Could you check a few things on this drawing? It's one solid part, dimensions in mm from its lowest x, y, z. A direction names the side the tool comes from. Give positions to 0.01 mm unless a question says otherwise; leave off trailing zeros. Loops run counter-clockwise (first coordinate to the right, second up) from the corner with the lowest first, then second, coordinate; pieces in that order, holes last. Notation, with made-up numbers: M -39.75,-10.5 L 4.25,-10.5 A11 ccw 4.25,9.5 Z; hole C -12,22 d4. An arc over 180 degrees is marked long. Answer as a JSON object with one key per item and string values.
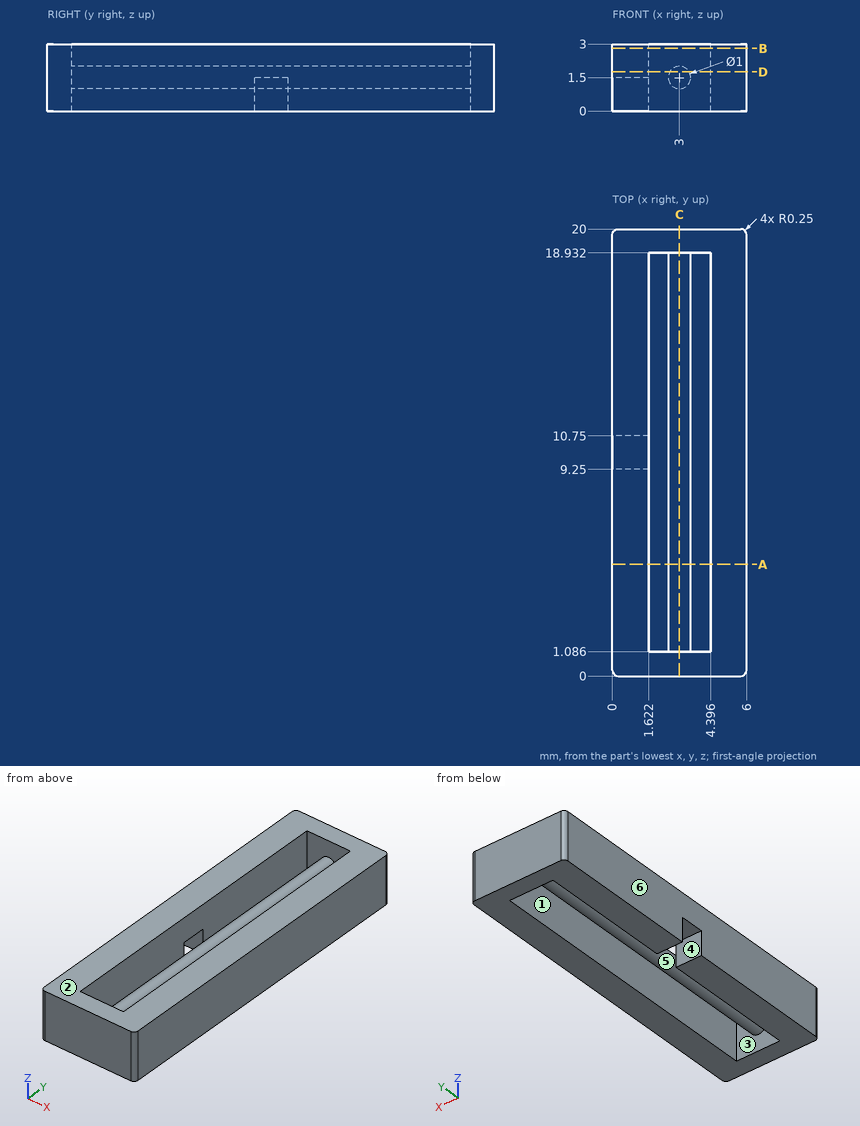
1) Suppose I cut it at C-C, the plane x = 3. Write out the boundary of the cut face in (y, z).
Answer list:
{"outline": "M 0,0 L 1.09,0 L 1.09,1 L 18.93,1 L 18.93,0 L 20,0 L 20,3 L 18.93,3 L 18.93,2 L 1.09,2 L 1.09,3 L 0,3 Z"}
2) Suppose I cut it at B-B, the plane z = 2.8. Write out the boundary of the cut face in (x, y).
Answer list:
{"outline": "M 0,0.25 A0.25 ccw 0.25,0 L 5.75,0 A0.25 ccw 6,0.25 L 6,19.75 A0.25 ccw 5.75,20 L 0.25,20 A0.25 ccw 0,19.75 Z; hole M 1.62,1.09 L 4.4,1.09 L 4.4,18.93 L 1.62,18.93 Z"}
3) If we mould it in two halves opening along X, with no side actions, what happens to the marked faces 4, 5 and 6? For each: +X half, -X half, draft (parallel to the pull), parting line (faces both ways), or undercut.
Answer list:
{"face 4": "draft", "face 5": "undercut", "face 6": "-X half"}
4) Please list where these lines run through material, in increasing order: line 1 along Y through (x, z) = (3.75, 1.4); line 2 along X through (y, z) = (1.5, 0.5); line 3 along X through (y, z) = (1.5, 1.85) (1 decimal). Write a range as from..to.
Answer list:
{"line 1": "0..1.09, 18.93..20", "line 2": "0..1.62, 4.4..6", "line 3": "0..1.6, 2.6..3.4, 4.4..6"}
5) Suppose I cut it at D-D, the plane z = 1.75. Write out the boundary of the cut face in (x, y).
Answer list:
{"outline": "M 0,0.25 A0.25 ccw 0.25,0 L 5.75,0 A0.25 ccw 6,0.25 L 6,19.75 A0.25 ccw 5.75,20 L 0.25,20 A0.25 ccw 0,19.75 Z; hole M 1.62,1.09 L 2.57,1.09 L 2.57,18.93 L 1.62,18.93 Z; hole M 3.43,1.09 L 4.4,1.09 L 4.4,18.93 L 3.43,18.93 Z"}
6) Will this pin go through, and if not, where does the flat tip stop? pin 1 Ø1.4 at (x, z) = (3.5, 1.5) entering from -Y.
Answer list:
{"pin 1": "y = 0"}
7) Suppose I cut it at A-A, the plane y = 5. Write out the boundary of the cut face in (x, z), and give its area (3 significant figures).
Answer list:
{"outline": "M 0,0 L 1.62,0 L 1.62,3 L 0,3 Z; C 3,1.5 d1; M 4.4,0 L 6,0 L 6,3 L 4.4,3 Z", "area": "10.5 mm^2"}
8) For the marked faces 1, 2 and 3, which set-ups out of +Z, -Z, +X, -X, +Y, -Y let a thin tool reach every point of the face, with its end or its side?
Answer list:
{"face 1": "+Z, -Z", "face 2": "+Z, +X, -X, +Y, -Y", "face 3": "none"}
